Build history of the part. All positions in model axes, mm. Face numbers are marked on the shaded views. A direction names the side the tool comes from. Round coordinates to 2 decimals unless told otherwise and drop trailing zeros. Loops run counter-clockwise (first coordinate to the right, second up) from the corner with the lowest first, then second, coordinate; pieces in that order, holes last.
Autodesk Inventor part; units mm, degrees
ref_plane "YZ Plane" through (0, 0, 0) normal (1, 0, 0) x (0, 1, 0)
ref_plane "XZ Plane" through (0, 0, 0) normal (0, 1, 0) x (-1, 0, 0)
ref_plane "XY Plane" through (0, 0, 0) normal (0, 0, 1) x (1, 0, 0)
sketch "Sketch1" plane through (0, 0, 0) normal (0, 0, 1) x (1, 0, 0)
  line L0 (-2.6984, 15.8681) -> (21.7216, 15.8681)
  line L1 (21.7216, 15.8681) -> (21.7216, -37.8319)
  line L2 (21.7216, -37.8319) -> (-2.6984, -37.8319)
  line L3 (-2.6984, -37.8319) -> (-2.6984, 15.8681)
  point P0 (0, 0)
  dimension "d0" = 53.7
  dimension "d1" = 24.42
extrude "Extrusion1" add sketch "Sketch1" along normal blind 2
sketch "Sketch2" plane through (0, 0, 2) normal (0, 0, 1) x (1, 0, 0)
  line L0 (-2.6984, -37.8319) -> (21.7216, -37.8319)
  line L1 (21.7216, 15.8681) -> (18.7216, 15.8681)
  line L2 (18.7216, 15.8681) -> (18.7216, -37.8319)
  line L3 (18.7216, -37.8319) -> (21.7216, -37.8319)
  line L4 (21.7216, -37.8319) -> (21.7216, 15.8681)
  line L5 (21.7216, -37.8319) -> (21.7216, 15.8681)
  line L6 (-2.6984, 15.8681) -> (21.7216, 15.8681)
  line L7 (21.7216, 15.8681) -> (21.7216, 12.8681)
  line L8 (21.7216, 12.8681) -> (-2.6984, 12.8681)
  line L9 (-2.6984, 12.8681) -> (-2.6984, 15.8681)
  line L10 (-2.6984, -37.8319) -> (21.7216, -37.8319)
  line L11 (21.7216, -37.8319) -> (21.7216, -34.8319)
  line L12 (21.7216, -34.8319) -> (-2.6984, -34.8319)
  line L13 (-2.6984, -34.8319) -> (-2.6984, -37.8319)
  point P0 (0, 0)
  dimension "d4" = 3
  dimension "d5" = 3
  dimension "d6" = 3
extrude "Extrusion2" add sketch "Sketch2" along normal blind 16
sketch "Sketch3" plane through (0, 0, 0) normal (0, 0, -1) x (-1, 0, 0)
  point P0 (0, 0)
sketch "Sketch4" plane through (0, 0, 0) normal (0, 0, -1) x (-1, 0, 0)
  circle A0 centre (-8.0116, 2.4017) radius 8.5
  circle A1 centre (-8.0116, -24.3699) radius 8.5
  line L0 (2.6984, -37.8319) -> (2.6984, 15.8681)
  line L1 (-21.7216, -37.8319) -> (2.6984, -37.8319)
  line L2 (2.6984, 15.8681) -> (-21.7216, 15.8681)
  line L3 (-18.7216, 12.8681) -> (-18.7216, -34.8319)
  point P0 (0, 0)
  dimension "d9" = 17
  dimension "d10" = 17
  dimension "d11" = 10.71
  dimension "d12" = 10.71
  dimension "d13" = 26.7716
  dimension "d14" = 13.462
  dimension "d15" = 13.4664
  dimension "d45" = 24.42
  dimension "d46" = 21.42
hole "Hole1" at (8.0116, 2.4017, 0) at (8.0116, -24.3699, 0) direction (0, 0, 1) diameter 17 depth 2 tip angle 118
sketch "Sketch5" plane through (0, 0, 2) normal (0, 0, 1) x (1, 0, 0)
  line L0 (-0.1076, -6.2299) -> (-2.6984, -6.2299)
  line L1 (-2.6984, -6.2299) -> (-2.6984, -15.7299)
  line L2 (-2.6984, -15.7299) -> (-0.1076, -15.7299)
  line L3 (-0.1076, -15.7299) -> (-0.1076, -6.2299)
  line L4 (21.7216, 15.8681) -> (-2.6984, 15.8681)
  line L5 (-2.6984, -37.8319) -> (21.7216, -37.8319)
  line L6 (-2.6984, 12.8681) -> (-2.6984, -34.8319)
  point P0 (0, 0)
  dimension "d23" = 9.5
  dimension "d24" = 22.098
  dimension "d25" = 22.102
  dimension "d26" = 2.5908
  dimension "d27" = 0
  dimension "d47" = 2.5908
extrude "Extrusion3" cut sketch "Sketch5" against normal blind 10
sketch "Sketch6" plane through (0, 0, 2) normal (0, 0, 1) x (1, 0, 0)
  line L0 (17.7216, -5.7319) -> (13.7216, -5.7319)
  line L1 (13.7216, -5.7319) -> (13.7216, -16.2319)
  line L2 (13.7216, -16.2319) -> (17.7216, -16.2319)
  line L3 (17.7216, -16.2319) -> (17.7216, -5.7319)
  line L4 (21.7216, 15.8681) -> (21.7216, -37.8319)
  line L5 (-2.6984, -37.8319) -> (21.7216, -37.8319)
  line L6 (21.7216, 15.8681) -> (-2.6984, 15.8681)
  point P0 (0, 0)
  dimension "d30" = 4
  dimension "d31" = 10.5
  dimension "d32" = 4
  dimension "d33" = 21.6
  dimension "d34" = 21.6
extrude "Extrusion4" cut sketch "Sketch6" against normal blind 10
sketch "Sketch7" plane through (-2.6984, 15.8681, 0) normal (0, 1, 0) x (1, 0, 0)
  line L0 (0, -2) -> (0, -18)
  line L1 (24.42, -18) -> (0, -18)
  line L2 (0, -18) -> (0, -16)
  line L3 (0, -16) -> (24.42, -16)
  line L4 (24.42, -16) -> (24.42, -18)
  point P0 (2.6984, 0)
  dimension "d37" = 2
extrude "Extrusion5" add sketch "Sketch7" along normal blind 4
sketch "Sketch8" plane through (21.7216, -37.8319, 0) normal (1, 0, 0) x (0, 0, -1)
  point P0 (0, 37.8319)
sketch "Sketch9" plane through (-2.6984, -37.8319, 0) normal (0, -1, 0) x (1, 0, 0)
  line L0 (24.42, 0) -> (24.42, 18)
  line L1 (0, 18) -> (24.42, 18)
  line L2 (24.42, 18) -> (24.42, 16)
  line L3 (24.42, 16) -> (0, 16)
  line L4 (0, 16) -> (0, 18)
  point P0 (2.6984, 0)
  dimension "d40" = 2
extrude "Extrusion6" add sketch "Sketch9" along normal blind 4
sketch "Sketch10" plane through (21.7216, -37.8319, 0) normal (1, 0, 0) x (0, 0, -1)
  line L0 (-18, -4) -> (-16, -4)
  line L1 (-16, -4) -> (-16, 57.7)
  line L2 (-16, 57.7) -> (-18, 57.7)
  line L3 (-18, 57.7) -> (-18, -4)
  point P0 (0, 37.8319)
extrude "Extrusion7" add sketch "Sketch10" along normal blind 4
equation "\"d11\" = 0.5 * d46"
equation "\"d12\" = 0.5 * d46"
equation "\"d33\" = d34"
properties part number "Sonar_Bracket" material "ABS Plastic"
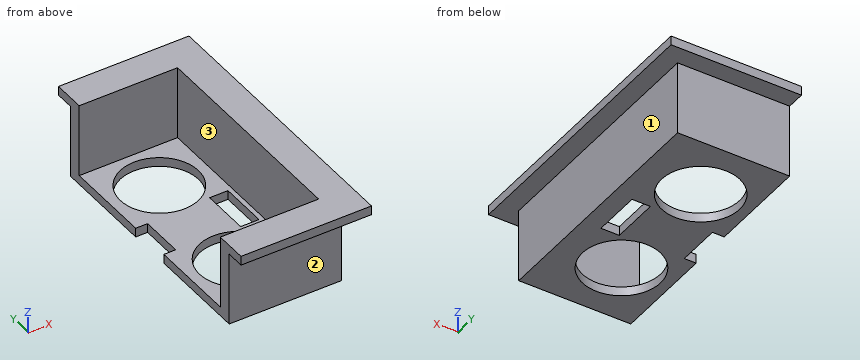
(1) Probe line 1 (Y direction, x = 6.25, z = 6.75); line 2 (Z direction, x = 17, y = -29.5); line 3 (Y direction, x = 21.25, z = 6.5). List the from-to ranges inside material, lowest first.
Responses:
line 1: y = -37.83 to -34.83, 12.87 to 15.87
line 2: z = 0 to 2
line 3: y = -37.83 to 15.87
(2) Slice it at D-D on x = 15.25. List the corners of the cut face in (y, z), plus the area to 3 significant figures.
Responses:
outline: (-41.83, 16) - (-37.83, 16) - (-37.83, 0) - (-28.83, 0) - (-28.83, 2) - (-34.83, 2) - (-34.83, 18) - (-41.83, 18) - close; (-19.91, 0) - (-16.23, 0) - (-16.23, 2) - (-19.91, 2) - close; (-5.73, 0) - (-2.05, 0) - (-2.05, 2) - (-5.73, 2) - close; (6.86, 0) - (15.87, 0) - (15.87, 16) - (19.87, 16) - (19.87, 18) - (12.87, 18) - (12.87, 2) - (6.86, 2) - close
area: 163 mm2
(3) Slice it at C-C on z = 14.5. List the corners of the cut face in (x, y), plus the area to 3 significant figures.
Responses:
outline: (-2.7, -37.83) - (21.72, -37.83) - (21.72, 15.87) - (-2.7, 15.87) - (-2.7, 12.87) - (18.72, 12.87) - (18.72, -34.83) - (-2.7, -34.83) - close
area: 290 mm2
(4) Which spindle directions (+Z, -Z, +X, -X, +Y, -Y) get a long thin tool onto all of the face, cutting with end or side? Do the marked faces 1, 2 and 3. Say none if no direction does.
Responses:
face 1: -Z, +X, +Y, -Y
face 2: -Z, +X, -X, -Y
face 3: +Z, -X
(5) Slice it at A-A on x = 11. List the corners of the cut face in (y, z).
Responses:
outline: (-41.83, 16) - (-37.83, 16) - (-37.83, 0) - (-32.33, 0) - (-32.33, 2) - (-34.83, 2) - (-34.83, 18) - (-41.83, 18) - close; (-16.41, 0) - (-5.56, 0) - (-5.56, 2) - (-16.41, 2) - close; (10.36, 0) - (15.87, 0) - (15.87, 16) - (19.87, 16) - (19.87, 18) - (12.87, 18) - (12.87, 2) - (10.36, 2) - close
(6) Slice it at B-B on y = 0.5. List the corners of the cut face in (x, z), plus the area to 3 significant figures.
Responses:
outline: (-2.7, 0) - (-0.27, 0) - (-0.27, 2) - (-2.7, 2) - close; (16.3, 0) - (21.72, 0) - (21.72, 16) - (25.72, 16) - (25.72, 18) - (18.72, 18) - (18.72, 2) - (16.3, 2) - close
area: 71.7 mm2
(7) Pin check, flat tips, straight feed: P1, Ø3, axis at y = -2, z = 10.5, coming from the +X side; P2, Ø8, axis at y = -22, z = 14.5, coming from the -X side; P3, Ø0.6, axis at y = -11.5, z = 0.5, coming from the -X side. Stop position of each tip, or through.
Responses:
P1: stops at x = 21.72
P2: stops at x = 18.72
P3: stops at x = -0.11
